Check sheet for the modelled part. Datum: model origin and axes. Units: mm. Round coordinates to 2 decimals unless told otherwise and drop trailing zeros. Order: outer loops, then holes, each group sorted by start corner. A loop starts at its lowest first (then second) coordinate and runs counter-clockwise, first axis right, second up.
Q1. Scan lines: probe 1 along X at (y, z) = (-15, -28.75); probe 2 along X at (y, z) = (-18, -24.5); probe 3 along X at (y, z) = (-18.5, -22.5). Record each from-to range of solid material in increasing order.
Q2. Depth check by flat-ended pin: P1, Ø10, axis at y = -3, z = -42.5, coming from the +X side; P2, Ø3, axis at x = -35.5, y = -22, coming from the -Z side; P3, Ø2, axis at x = -53, z = -32, coming from the +Y side; P4, Ø3, axis at x = 7.5, z = -39.49, coming from the +Y side. Enter the tip coordinate at first touch or a pass-through.
Q3. Cross-section at A-A on z = -33.5. Record the cut outline in (x, y).
Q4. Cross-section at C-C on y = -19. Record the cut outline in (x, z).
Q5. Mould release check, pull along X, two halves, no side actions. Record for faces 1 (the cylindrical face through (-18.13, -22.345, -42.59)), 2 (the cylindrical face through (16.86, -12.88, -41.25)), 3 (the cylindrical face through (7.07, -12.53, -25.44)): +X half, -X half, draft (parallel to the pull), parting line (faces both ways), or undercut.
Q6. Cross-section at D-D on y = -23.5. Record the cut outline in (x, z), then the cut area to 3 significant figures.
Q7. Cross-section at B-B on x = -45. Record the cut outline in (y, z) (3 decimals), then the cut area to 3 significant figures.
from build123d import *

# Parameters (mm, degrees)
F0_W     = 85
F0_H     = 28
F1_DEPTH = 25.4
F2_R     = 10.16
F4_DEPTH = 25.4
F5_R     = 2
F7_DEPTH = 35


with BuildPart() as f1:
    # F0 (on Front) → F1 (new body)
    with BuildSketch(Plane.XZ):
        with Locations((-23.7341526002, -31.4873820276)):
            Rectangle(F0_W, F0_H)
    extrude(amount=F1_DEPTH)

    # F2
    f2_edges = [f1.edges().sort_by_distance(p)[0] for p in [
        (-66.234153, -12.7, -17.487382),
        (-66.234153, -12.7, -45.487382),
        (-66.234153, 0, -31.487382),
        (-66.234153, -25.4, -31.487382),
        (18.765847, -12.7, -17.487382),
        (-23.734153, 0, -17.487382),
        (-23.734153, -25.4, -17.487382),
        (18.765847, -12.7, -45.487382),
        (-23.734153, 0, -45.487382),
        (-23.734153, -25.4, -45.487382),
    ]]
    fillet(f2_edges, radius=F2_R)

    # F3 (on face) → F4 (cut)
    with BuildSketch(Plane(origin=(0, 0, 0), x_dir=(-1, 0, 0), z_dir=(0, 1, 0))):
        with BuildLine():
            Line((37.2422865066, -27.6473820276), (50.4459766734, -27.6473820276))
            ThreePointArc((50.4459766734, -27.6473820276), (43.84413159, -21.7962196174), (37.2422865066, -27.6473820276))
        make_face()
        with BuildLine():
            ThreePointArc((37.2422865066, -27.6473820276), (43.4439877437, -35.0841699714), (50.49413159, -28.4462196174))
            ThreePointArc((50.49413159, -28.4462196174), (50.482081944, -28.0460757711), (50.4459766734, -27.6473820276))
            Line((50.4459766734, -27.6473820276), (37.2422865066, -27.6473820276))
        make_face()
    extrude(amount=-F4_DEPTH, mode=Mode.SUBTRACT)

    # F5 (on Front) → F7 (cut)
    with BuildSketch(Plane.XZ):
        with Locations((7.5045232661, -23.4873820276)):
            Circle(F5_R)
        with Locations((7.5045232661, -39.4873820276)):
            Circle(F5_R)
    extrude(amount=F7_DEPTH, mode=Mode.SUBTRACT)


solid = f1.part
Results found:
1. probe 1: x = -66.23 to -50.49, -37.2 to 18.77
1. probe 2: x = -65.33 to -49.2, -38.49 to 5.78, 9.23 to 18.27
1. probe 3: x = -64.2 to -46.82, -40.87 to 5.77, 9.24 to 17.37
2. P1: stops at x = 18.53
2. P2: stops at z = -44.02
2. P3: stops at y = 0
2. P4: passes through
3. outline: (-66.23, -15.24) arc R10.16 ccw to (-56.07, -25.4) - (-48.17, -25.4) - (-48.17, 0) - (-56.07, 0) arc R10.16 ccw to (-66.23, -10.16) - close; (-39.52, -25.4) - (18.77, -25.4) - (18.77, 0) - (-39.52, 0) - close
4. outline: (-65.51, -35.33) arc R9.44 ccw to (-56.07, -44.77) - (12.37, -44.77) arc R10.16 ccw to (18.77, -35.33) - (18.77, -27.65) arc R10.16 ccw to (12.37, -18.21) - (-56.07, -18.21) arc R9.44 ccw to (-65.51, -27.65) - close; hole circle Ø13.3 at (-43.84, -28.45); hole circle Ø4 at (7.5, -39.49); hole circle Ø4 at (7.5, -23.49)
5. face 1: draft
5. face 2: +X half
5. face 3: undercut
6. outline: (-61.99, -35.33) arc R5.92 ccw to (-56.07, -41.24) - (6.55, -41.24) arc R2 cw (long way) to (8.46, -41.24) - (16.87, -41.24) arc R10.16 ccw to (18.77, -35.33) - (18.77, -27.65) arc R10.16 ccw to (16.87, -21.73) - (8.46, -21.73) arc R2 cw (long way) to (6.55, -21.73) - (-56.07, -21.73) arc R5.92 ccw to (-61.99, -27.65) - close; hole circle Ø13.3 at (-43.84, -28.45)
6. area: 1,390 mm2
7. outline: (-25.4, -35.327) arc R10.16 ccw to (-15.24, -45.487) - (-10.16, -45.487) arc R10.16 ccw to (0, -35.327) - (0, -34.995) - (-25.4, -34.995) - close; (-23.616, -21.897) - (-1.784, -21.897) arc R10.16 ccw to (-10.16, -17.487) - (-15.24, -17.487) arc R10.16 ccw to start
7. area: 296 mm2
